CAD build for the part. Positions are in the model's coordinates, mm. Coordinates: 2 decimals unless noted, no trailing zeros. Order: outer loops, then holes, each group sorted by start corner. A loop starts at its lowest first (then second) coordinate and runs counter-clockwise, first axis right, second up. Notation, with made-up numbers: (6, 42) - (60, 42) arc R6 cw to (60, 46) - close; hole circle Ø2 at (27.25, 11.5). An arc over 180 degrees is marked (long way). Return JSON: item names as keys, results as strings.
from build123d import *

# Parameters (mm, degrees)
ESQUISSE1_W        = 180.86
ESQUISSE1_H        = 273
ESQUISSE1_R        = 1.5
ESQUISSE1_W_2      = 52
ESQUISSE1_H_2      = 28
ESQUISSE1_W_3      = 126
ESQUISSE1_H_3      = 40
BOSS_EXTRU_1_DEPTH = 4
D_GAGEMENT_M31_D   = 3.4
CONG_1_R           = 3


with BuildPart() as part:
    # Esquisse1 → Boss.-Extru.1 (new body)
    with BuildSketch(Plane.XY):
        with Locations((90.43, 136.5)):
            Rectangle(ESQUISSE1_W, ESQUISSE1_H)
        with Locations((30.43, 236.5)):
            Circle(ESQUISSE1_R, mode=Mode.SUBTRACT)
        with Locations((150.43, 236.5)):
            Circle(ESQUISSE1_R, mode=Mode.SUBTRACT)
        with Locations((30.43, 70.5)):
            Circle(ESQUISSE1_R, mode=Mode.SUBTRACT)
        with Locations((150.43, 70.5)):
            Circle(ESQUISSE1_R, mode=Mode.SUBTRACT)
        with Locations((90.43, 56)):
            Rectangle(ESQUISSE1_W_2, ESQUISSE1_H_2, mode=Mode.SUBTRACT)
        with Locations((90.93, 124)):
            Rectangle(ESQUISSE1_W_3, ESQUISSE1_H_3, mode=Mode.SUBTRACT)
    extrude(amount=BOSS_EXTRU_1_DEPTH)

    # Dégagement M31 (through all)
    with Locations(Plane.XY.offset(4)):
        with Locations((30.43, 236.5), (150.43, 236.5), (150.43, 70.5), (30.43, 70.5)):
            Hole(D_GAGEMENT_M31_D / 2)

    # Congé1
    cong_1_edges = [part.edges().sort_by_distance(p)[0] for p in [
        (64.43, 70, 2),
        (64.43, 42, 2),
        (116.43, 42, 2),
        (116.43, 70, 2),
        (27.93, 144, 2),
        (27.93, 104, 2),
        (153.93, 104, 2),
        (153.93, 144, 2),
        (0, 273, 2),
        (180.86, 273, 2),
        (180.86, 0, 2),
        (0, 0, 2),
    ]]
    fillet(cong_1_edges, radius=CONG_1_R)


solid = part.part
Item 1: Band-saw the part on D-D, the plane x = 85.5. List the corners of the cut face in (y, z), then the cut area to 3 significant figures.
Findings below:
{"outline": "(0, 0) - (42, 0) - (42, 4) - (0, 4) - close; (70, 0) - (104, 0) - (104, 4) - (70, 4) - close; (144, 0) - (273, 0) - (273, 4) - (144, 4) - close", "area": "820 mm²"}
Item 2: Band-saw the part on B-B, the plane x = 52.5. List the corners of the cut face in (y, z), then the cut area to 3 significant figures.
Findings below:
{"outline": "(0, 0) - (104, 0) - (104, 4) - (0, 4) - close; (144, 0) - (273, 0) - (273, 4) - (144, 4) - close", "area": "932 mm²"}
Item 3: Drop a flat-ended pin along its axis: P1, Ø4, axis at x = 30.43, y = 70.5, coming from the +Z side. Give the stop position or say it passes through.
Findings below:
{"P1": "stops at z = 4"}
Item 4: Wall check: L1, parallel to Y at x = 106, z = 3.8; L2, parallel to X at y = 70.5, z = 3.2; L3, parallel to Y at x = 150.43, z = 2.05. Give the ranges that are in metal, low to high. Write a range as [from, to].
Findings below:
{"L1": "y = [0, 42], [70, 104], [144, 273]", "L2": "x = [0, 28.73], [32.13, 148.73], [152.13, 180.86]", "L3": "y = [0, 68.8], [72.2, 104], [144, 234.8], [238.2, 273]"}
Item 5: Band-saw the part on A-A, the plane y = 124.5. List the corners of the cut face in (x, z), then the cut area to 3 significant figures.
Findings below:
{"outline": "(0, 0) - (27.93, 0) - (27.93, 4) - (0, 4) - close; (153.93, 0) - (180.86, 0) - (180.86, 4) - (153.93, 4) - close", "area": "219 mm²"}
Item 6: Band-saw the part on C-C, the plane z = 1.1. List the corners of the cut face in (x, y), then the cut area to 3 significant figures.
Findings below:
{"outline": "(0, 3) arc R3 ccw to (3, 0) - (177.86, 0) arc R3 ccw to (180.86, 3) - (180.86, 270) arc R3 ccw to (177.86, 273) - (3, 273) arc R3 ccw to (0, 270) - close; hole (27.93, 107) arc R3 ccw to (30.93, 104) - (150.93, 104) arc R3 ccw to (153.93, 107) - (153.93, 141) arc R3 ccw to (150.93, 144) - (30.93, 144) arc R3 ccw to (27.93, 141) - close; hole circle Ø3.4 at (30.43, 70.5); hole circle Ø3.4 at (30.43, 236.5); hole (64.43, 45) arc R3 ccw to (67.43, 42) - (113.43, 42) arc R3 ccw to (116.43, 45) - (116.43, 67) arc R3 ccw to (113.43, 70) - (67.43, 70) arc R3 ccw to (64.43, 67) - close; hole circle Ø3.4 at (150.43, 70.5); hole circle Ø3.4 at (150.43, 236.5)", "area": "42,900 mm²"}
